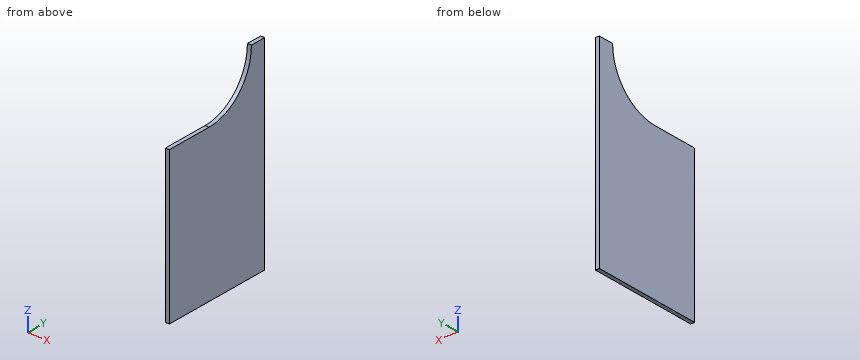
from build123d import *

# Parameters (mm, degrees)
BOSS_EXTRUDE1_DEPTH = 6.35


with BuildPart() as part:
    # Sketch1 → Boss-Extrude1 (new body)
    with BuildSketch(Plane(origin=(0, 0, 0), x_dir=(0, 0, -1), z_dir=(1, 0, 0))):
        with BuildLine():
            Line((0, 0), (0, 75))
            ThreePointArc((0, 75), (-23.431457505, 131.568542495), (-80, 155))
            Line((-80, 155), (-80, 180))
            Line((-80, 180), (240, 180))
            Line((240, 180), (240, 0))
            Line((240, 0), (0, 0))
        make_face()
    extrude(amount=BOSS_EXTRUDE1_DEPTH)


solid = part.part
Work out the finished part from the listing and answer in its coordinate system (mm). Give positions to 0.01 mm unless a question says otherwise; leave off trailing zeros. Loops run counter-clockwise (first coordinate to the right, second up) from the corner with the lowest first, then second, coordinate; pieces in that order, holes last. Notation, with made-up numbers: (67.25, -32.75) -> (105.25, -32.75) arc R31 cw to (105.25, -6.75) -> close; hole circle Ø8 at (-29.75, -5). An arc over 180 degrees is marked (long way). Use a Markdown table: item, result. Add a question column.
1. Flat-ended cylindrical pins translate along their axes: pin 1 Ø1.9 at (x, y) = (4, 40) entering from +Z; pin 2 Ø1.5 at (y, z) = (109.5, -8.5) entering from -X. Find the tip coordinate at first contact, or state that the pin passes through.
2. Section A-A on x = 4 is taken. Determine the outline of the cut face in (y, z), and give its area (3 significant figures).
3. Section C-C on y = 35.5 is taken. Determine the outline of the cut face in (x, z), and give its area (3 significant figures).
4. Find the intervals of material crossed by probe 1 along Z at (x, y) = (4.5, 26); probe 2 along Z at (x, y) = (3.5, 120); probe 3 along Y at (x, z) = (2.75, 19.5), in increasing order.
5. Section B-B on z = 52 is taken. Determine the outline of the cut face in (x, y).
Results below:
| question | item | result |
|---|---|---|
| 1 | pin 1 | stops at z = 0 |
| 1 | pin 2 | stops at x = 0 |
| 2 | outline | (0, -240) -> (180, -240) -> (180, 80) -> (155, 80) arc R80 cw to (75, 0) -> (0, 0) -> close |
| 2 | area | 46,600 mm^2 |
| 3 | outline | (0, -240) -> (6.35, -240) -> (6.35, 0) -> (0, 0) -> close |
| 3 | area | 1,520 mm^2 |
| 4 | probe 1 | z = -240 to 0 |
| 4 | probe 2 | z = -240 to 13.86 |
| 4 | probe 3 | y = 127.34 to 180 |
| 5 | outline | (0, 149.94) -> (6.35, 149.94) -> (6.35, 180) -> (0, 180) -> close |
